from build123d import *

# Parameters (mm, degrees)
BOSS_EXTRUDE1_DEPTH      = 100
BOSS_EXTRUDE1_DEPTH_BACK = 100
CHAMFER1_SIZE            = 0.21
CUT_EXTRUDE1_DEPTH       = 101.488805347
CUT_EXTRUDE1_DEPTH_BACK  = 101.488805347
SKETCH4_W                = 104.931235955
SKETCH4_H                = 144.2275


with BuildPart() as part:
    # Sketch3 → Boss-Extrude1 (new, two sides: drawn at the far end of the back side and taken through both)
    with BuildSketch(Plane.XY.offset(-BOSS_EXTRUDE1_DEPTH_BACK)):
        with BuildLine():
            Line((-2.5, 4), (-2.5, 6.538348415))
            ThreePointArc((-2.5, 6.538348415), (0, -7), (2.5, 6.538348415))
            Line((2.5, 6.538348415), (2.5, 4))
            Line((2.5, 4), (-2.5, 4))
        make_face()
    extrude(amount=BOSS_EXTRUDE1_DEPTH + BOSS_EXTRUDE1_DEPTH_BACK)

    # Chamfer1
    chamfer1_edges = [part.edges().sort_by_distance(p)[0] for p in [
        (0, -7, -100),
        (0, -7, 100),
    ]]
    chamfer(chamfer1_edges, length=CHAMFER1_SIZE)

    # Sketch4 → Cut-Extrude1 (cut, two sides: drawn at the far end of the back side and taken through both)
    with BuildSketch(Plane(origin=(0, 0, 0), x_dir=(1, 0, 0), z_dir=(0, 1, 0)).offset(-CUT_EXTRUDE1_DEPTH_BACK)):
        with Locations((22.551011235, 27.88625)):
            Rectangle(SKETCH4_W, SKETCH4_H)
    extrude(amount=CUT_EXTRUDE1_DEPTH + CUT_EXTRUDE1_DEPTH_BACK, mode=Mode.SUBTRACT)


solid = part.part
CAD build for the part. Positions are in the model's coordinates, mm. A direction names the side the tool comes from. Coordinates: 2 decimals unless noted, no trailing zeros. Loops run counter-clockwise (first coordinate to the right, second up) from the corner with the lowest first, then second, coordinate; pieces in that order, holes last. Notation, with made-up numbers: (20, -40) - (73, -40) arc R20 cw to (73, -18) - close; hole circle Ø5 at (81, -2.5). An arc over 180 degrees is marked (long way). Use one line per item in the form item = value. Start each with the question number.
1) Drill centre lines: L1, parallel to X at y = 1.75, z = 86; L2, parallel to X at y = 4.25, z = 50; L3, parallel to X at y = 5, z = 53.5. Where is each one in solid material? Low to high. Write a range as from..to.
2) Band-saw the part on B-B (z = 81). Give the cut face in (x, y), and give its area (3 significant figures).
3) Flat gauge pins, fed straight in: pin 1 (8 mm diameter, centred on x = 3, z = 73.5, fed in from +Y); pin 2 (3 mm diameter, centred on y = 4.5, z = 83, fed in from +X); pin 3 (1 mm diameter, centred on y = -2, z = 66.5, fed in from +X). Where does each tip first touch, or does it go through?
4) Tool access for faces 5 (the face through (0, 0, 100)), 6 (the face through (0, 4, 72)): list every direction of +Z, -Z, +X, -X, +Y, -Y with a clear straight run to the whole face (end or side of a thin tool).
5) Band-saw the part on A-A (x = 0). Give the cut face in (y, z), and give its area (3 significant figures).
6) Two-plate mould, pull along X, no slides. Class faces 1 (the face through (0, 0, 44.227)), 2 (the face through (2.5, 5, 72)), 3 (the face through (-2.5, 5, 72)), 4 (the face through (0, -7, 72)): +X half, -X half, draft (parallel to the pull), parting line (faces both ways), or undercut.
Check values:
q1.L1 = -6.78..6.78
q1.L2 = -5.56..-2.5, 2.5..5.56
q1.L3 = -4.9..-2.5, 2.5..4.9
q2.outline = (-2.5, 4) - (-2.5, 6.54) arc R7 ccw (long way) to (2.5, 6.54) - (2.5, 4) - close
q2.area = 140 mm2
q3.pin_1 = 6.54
q3.pin_2 = 6.32
q3.pin_3 = 6.84
q4.face_5 = +Z, +X, -X, +Y, -Y
q4.face_6 = +Z, -Z, +Y
q5.outline = (-7, 44.23) - (4, 44.23) - (4, 100) - (-6.79, 100) - (-7, 99.79) - close
q5.area = 613 mm2
q6.face_1 = draft
q6.face_2 = undercut
q6.face_3 = undercut
q6.face_4 = parting line
